```python
from build123d import *

# Parameters (mm, degrees)
SKETCH1_R                = 140
BOSS_EXTRUDE1_DEPTH      = 225
SKETCH2_R                = 99
CUT_EXTRUDE1_DEPTH       = 300.708191413
BOSS_EXTRUDE2_START      = -32
BOSS_EXTRUDE2_DEPTH      = 32
CIRPATTERN1_COUNT        = 3
CIRPATTERN2_START        = -32
CIRPATTERN2_COPY_1_DEPTH = 32
CIRPATTERN2_COPY_2_DEPTH = 32
CIRPATTERN2_COPY_3_DEPTH = 32
CIRPATTERN2_COPY_4_DEPTH = 32
BOSS_EXTRUDE3_REACH      = 491.361
BOSS_EXTRUDE3_END_RADIUS = 140
SKETCH5_R                = 100
SKETCH6_R                = 50
CUT_EXTRUDE2_DEPTH       = 25
SKETCH9_R                = 28
CUT_EXTRUDE3_DEPTH       = 490.361006427
SKETCH11_R               = 12
CUT_EXTRUDE4_DEPTH       = 15
CIRPATTERN4_COUNT        = 3


with BuildPart() as part:
    # Sketch1 → Boss-Extrude1 (new body)
    with BuildSketch(Plane(origin=(0, 0, 0), x_dir=(1, 0, 0), z_dir=(0, 1, 0))):
        with Locations(Location((0, 0, 0), (0, 0, 270))):
            Circle(SKETCH1_R)
    extrude(amount=BOSS_EXTRUDE1_DEPTH)

    # Sketch2 → Cut-Extrude1 (cut, through all)
    with BuildSketch(Plane(origin=(0, 225, 0), x_dir=(1, 0, 0), z_dir=(0, 1, 0))):
        with Locations(Location((0, 0, 0), (0, 0, 270))):
            Circle(SKETCH2_R)
    extrude(amount=-CUT_EXTRUDE1_DEPTH, mode=Mode.SUBTRACT)

    # Sketch3 → Boss-Extrude2 (add)
    with BuildSketch(Plane(origin=(0, 225, 0), x_dir=(1, 0, 0), z_dir=(0, 1, 0)).offset(BOSS_EXTRUDE2_START)):
        with BuildLine():
            ThreePointArc((50, 175), (0, 225), (-50, 175))
            Line((-50, 175), (-50, 130.766968306))
            ThreePointArc((-50, 130.766968306), (0, 140), (50, 130.766968306))
            Line((50, 130.766968306), (50, 175))
        make_face()
        with BuildLine():
            ThreePointArc((-23.5, 175), (0, 198.5), (23.5, 175))
            ThreePointArc((23.5, 175), (0, 151.5), (-23.5, 175))
        make_face(mode=Mode.SUBTRACT)
    boss_extrude2 = extrude(amount=BOSS_EXTRUDE2_DEPTH)

    # CirPattern1: Boss-Extrude2 ×3 about axis
    cirpattern1_axis = Axis((0, 0, 0), (0, 1, 0))
    for i in range(1, CIRPATTERN1_COUNT):
        add(boss_extrude2.rotate(cirpattern1_axis, i * 360 / CIRPATTERN1_COUNT))

    # Mirror3: Boss-Extrude2 across plane
    add(boss_extrude2.mirror(Plane(origin=(0, 112.5, 0), x_dir=(0, 0, 1), z_dir=(0, -1, 0))))

    # CirPattern2 copy 1 sketch → CirPattern2 copy 1 (add)
    with BuildSketch(Plane(origin=(0, 0, 0), x_dir=(-0.4999999999999998, 0, 0.8660254037844387), z_dir=(0, -1, 0)).offset(CIRPATTERN2_START)):
        with BuildLine():
            ThreePointArc((50, -175), (0, -225), (-50, -175))
            Line((-50, -175), (-50, -130.766968306))
            ThreePointArc((-50, -130.766968306), (0, -140), (50, -130.766968306))
            Line((50, -130.766968306), (50, -175))
        make_face()
        with BuildLine():
            ThreePointArc((-23.5, -175), (0, -198.5), (23.5, -175))
            ThreePointArc((23.5, -175), (0, -151.5), (-23.5, -175))
        make_face(mode=Mode.SUBTRACT)
    extrude(amount=CIRPATTERN2_COPY_1_DEPTH)

    # CirPattern2 copy 2 sketch → CirPattern2 copy 2 (add)
    with BuildSketch(Plane(origin=(0, 0, 0), x_dir=(-0.5000000000000004, 0, -0.8660254037844384), z_dir=(0, -1, 0)).offset(CIRPATTERN2_START)):
        with BuildLine():
            ThreePointArc((50, -175), (0, -225), (-50, -175))
            Line((-50, -175), (-50, -130.766968306))
            ThreePointArc((-50, -130.766968306), (0, -140), (50, -130.766968306))
            Line((50, -130.766968306), (50, -175))
        make_face()
        with BuildLine():
            ThreePointArc((-23.5, -175), (0, -198.5), (23.5, -175))
            ThreePointArc((23.5, -175), (0, -151.5), (-23.5, -175))
        make_face(mode=Mode.SUBTRACT)
    extrude(amount=CIRPATTERN2_COPY_2_DEPTH)

    # CirPattern2 copy 3 sketch → CirPattern2 copy 3 (add)
    with BuildSketch(Plane(origin=(0, 225, 0), x_dir=(-0.4999999999999998, 0, 0.8660254037844387), z_dir=(0, 1, 0)).offset(CIRPATTERN2_START)):
        with BuildLine():
            ThreePointArc((50, 175), (0, 225), (-50, 175))
            Line((-50, 175), (-50, 130.766968306))
            ThreePointArc((-50, 130.766968306), (0, 140), (50, 130.766968306))
            Line((50, 130.766968306), (50, 175))
        make_face()
        with BuildLine():
            ThreePointArc((-23.5, 175), (0, 198.5), (23.5, 175))
            ThreePointArc((23.5, 175), (0, 151.5), (-23.5, 175))
        make_face(mode=Mode.SUBTRACT)
    extrude(amount=CIRPATTERN2_COPY_3_DEPTH)

    # CirPattern2 copy 4 sketch → CirPattern2 copy 4 (add)
    with BuildSketch(Plane(origin=(0, 225, 0), x_dir=(-0.5000000000000004, 0, -0.8660254037844384), z_dir=(0, 1, 0)).offset(CIRPATTERN2_START)):
        with BuildLine():
            ThreePointArc((50, 175), (0, 225), (-50, 175))
            Line((-50, 175), (-50, 130.766968306))
            ThreePointArc((-50, 130.766968306), (0, 140), (50, 130.766968306))
            Line((50, 130.766968306), (50, 175))
        make_face()
        with BuildLine():
            ThreePointArc((-23.5, 175), (0, 198.5), (23.5, 175))
            ThreePointArc((23.5, 175), (0, 151.5), (-23.5, 175))
        make_face(mode=Mode.SUBTRACT)
    extrude(amount=CIRPATTERN2_COPY_4_DEPTH)

    # Boss-Extrude3: up to this cylinder (the profile starts outside it)
    boss_extrude3_end = Plane(origin=(0, 109.390064, 0), z_dir=(0, -1, 0)) * Cylinder(BOSS_EXTRUDE3_END_RADIUS, 1263.722, mode=Mode.PRIVATE)
    # Sketch5 → Boss-Extrude3 (add, up to the surface)
    with BuildSketch(Plane.XY.offset(160), mode=Mode.PRIVATE) as boss_extrude3_sk1:
        with Locations((0, 109.390064354)):
            Circle(SKETCH5_R)
    boss_extrude3_tool1 = extrude(boss_extrude3_sk1.sketch, amount=-BOSS_EXTRUDE3_REACH, mode=Mode.PRIVATE) - boss_extrude3_end
    add(boss_extrude3_tool1.solids().sort_by_distance((0, 109.390064, 160))[0])

    # Sketch6 → Cut-Extrude2 (cut)
    with BuildSketch(Plane.XY.offset(160)):
        with Locations((0, 109.390064354)):
            Circle(SKETCH6_R)
    extrude(amount=-CUT_EXTRUDE2_DEPTH, mode=Mode.SUBTRACT)

    # Sketch9 → Cut-Extrude3 (cut, through all)
    with BuildSketch(Plane.XY.offset(160)):
        with Locations((0, 109.390064354)):
            Circle(SKETCH9_R)
    extrude(amount=-CUT_EXTRUDE3_DEPTH, mode=Mode.SUBTRACT)

    # Sketch11 → Cut-Extrude4 (cut)
    with BuildSketch(Plane.XY.offset(160)):
        with Locations((0, 184.390064354)):
            Circle(SKETCH11_R)
    cut_extrude4 = extrude(amount=-CUT_EXTRUDE4_DEPTH, mode=Mode.SUBTRACT)

    # CirPattern4: Cut-Extrude4 ×3 about axis
    cirpattern4_axis = Axis((0, 109.390064354, 0), (0, 0, 1))
    for i in range(1, CIRPATTERN4_COUNT):
        add(cut_extrude4.rotate(cirpattern4_axis, i * 360 / CIRPATTERN4_COUNT), mode=Mode.SUBTRACT)


solid = part.part
```
Geometry check sheet. Reference: the model listing, model coordinates, mm. A direction names the side the tool comes from. Round coordinates to 2 decimals unless told otherwise and drop trailing zeros. Loops run counter-clockwise (first coordinate to the right, second up) from the corner with the lowest first, then second, coordinate; pieces in that order, holes last. Notation, with made-up numbers: M -8.75,3.5 L 8.25,3.5 A16 ccw 8.25,8.5 Z; hole C 34,-15.75 d6. An arc over 180 degrees is marked long. Return JSON: item names as keys, results as strings. Group by question number.
(1) Scan lines: line 1 along Y through (x, z) = (0, 154.75); line 2 along Z through (x, y) = (0, 204.5); line 3 along X through (y, z) = (17, 87). Record each from-to range of solid material in increasing order. Write a range as [from, to].
(2) Section check D-D, the plane z = 87.5. Give the number of separate pieces and of enclosed holes in the cut face, and give its area (3 significant figures).
(3) Section check A-A, the plane z = 0. Enter the section's corners in (x, y), and give its area (4 significant figures).
(4) Section check C-C, the plane y = 69. Enter the section's corners in (x, z), and give its area (3 significant figures).
(5) Set-up check for faces 1 (the face through (50, 16, -153)), 2 (the face through (177, 32, 90)), 3 (the face through (-172, 193, 100)): record each of +Z, -Z, +X, -X, +Y, -Y from which the full face is reachable in a straight line by a thin tool's end or side.
(6) Mould release check, pull along Y, two halves, no side actions. Record for faces 4 (the face through (63.39, 83.788, 152.605)), 5 (the face through (-195.395, 16.224, 111.542)): pulls with the +Y half, pulls with the -Y half, needs draft (parallel to the pull), parting line crosses it, or undercut.
(7) Section check B-B, the plane x = 161.5. Enter the section's corners in (y, z), and give its area (3 significant figures).
(8) Go/stop test with flat-tipped pins: pin 1 (12 mm diameter, centred on x = 136.5, z = -6, fed in from -Y); pin 2 (2 mm diameter, centred on x = 143.5, y = 196, fed in from -Z); pin 3 (3 mm diameter, centred on y = 161.5, z = 64.5, fed in from -X); pin 4 (9.5 mm diameter, centred on y = 14, z = -158, fed in from -X). Record where each tip stops, or that it passes through.
Data:
{
 "1": {"line 1": "[9.39, 59.39], [159.39, 172.39], [196.39, 209.39]", "line 2": "[-225, -198.5], [-151.5, -99], [99, 160]", "line 3": "[-201.55, -175.05], [-128.06, -47.24], [47.24, 128.06], [175.05, 201.55]"},
 "2": {"separate pieces": "6", "enclosed holes": "0", "area": "34,100 mm²"},
 "3": {"outline": "M -140,0 L -99,0 L -99,225 L -140,225 Z; M 99,0 L 140,0 L 140,225 L 99,225 Z", "area": "18,450 mm²"},
 "4": {"outline": "M -91.48,105.98 A140 ccw long 91.48,105.98 L 91.48,160 L 76.6,160 L 76.6,145 L 53.31,145 L 53.31,160 L 29.47,160 L 29.47,135 L -29.47,135 L -29.47,160 L -53.31,160 L -53.31,145 L -76.6,145 L -76.6,160 L -91.48,160 Z; hole C 0,0 d198", "area": "34,200 mm²"},
 "5": {"face 1": "-Z, +X, +Y, -Y", "face 2": "+Z, +X", "face 3": "+Z, -X"},
 "6": {"face 4": "undercut", "face 5": "needs draft"},
 "7": {"outline": "M 0,35.51 L 32,35.51 L 32,66.21 L 0,66.21 Z; M 0,108.79 L 32,108.79 L 32,136.5 L 0,136.5 Z; M 193,35.51 L 225,35.51 L 225,66.21 L 193,66.21 Z; M 193,108.79 L 225,108.79 L 225,136.5 L 193,136.5 Z", "area": "3,740 mm²"},
 "8": {"pin 1": "y = 0", "pin 2": "z = 24.54", "pin 3": "x = -125.02", "pin 4": "x = -50"}
}
